```python
from build123d import *

# Parameters (mm, degrees)
SKETCH1_R           = 6.25
BOSS_EXTRUDE1_DEPTH = 8
BOSS_EXTRUDE1_DRAFT = -3
BOSS_EXTRUDE2_DEPTH = 4.5
SKETCH3_R           = 5
BOSS_EXTRUDE3_DEPTH = 2
SKETCH9_R           = 3.5
BOSS_EXTRUDE6_DEPTH = 0.5
FILLET1_R           = 1
SKETCH4_R           = 3
BOSS_EXTRUDE4_DEPTH = 1
SKETCH5_R           = 5
BOSS_EXTRUDE5_DEPTH = 2
SKETCH6_R           = 2
CUT_EXTRUDE1_DEPTH  = 9.5
CUT_EXTRUDE2_DEPTH  = 6.5
SKETCH8_R           = 4.5
CUT_EXTRUDE3_DEPTH  = 2


with BuildPart() as part:
    # Sketch1 → Boss-Extrude1 (with draft: the straight prism first)
    with BuildSketch(Plane.XY):
        Circle(SKETCH1_R)
    extrude(amount=BOSS_EXTRUDE1_DEPTH)
    # Boss-Extrude1: the draft: its side faces are tilted about the plane it starts from
    boss_extrude1_sides = [part.faces().sort_by_distance(p)[0] for p in [
        (-6.25, 0, 4),
    ]]
    draft(boss_extrude1_sides, Plane.XY, BOSS_EXTRUDE1_DRAFT)

    # Sketch2 → Boss-Extrude2 (add)
    with BuildSketch(Plane.XY.offset(8)):
        Polygon((8.082903769, 0), (4.041451884, 7), (-4.041451884, 7), (-8.082903769, 0), (-4.041451884, -7), (4.041451884, -7), align=None)
    extrude(amount=BOSS_EXTRUDE2_DEPTH)

    # Sketch3 → Boss-Extrude3 (add)
    with BuildSketch(Plane.XY.offset(12.5)):
        Circle(SKETCH3_R)
    extrude(amount=BOSS_EXTRUDE3_DEPTH)

    # Sketch9 → Boss-Extrude6 (add)
    with BuildSketch(Plane.XY.offset(14.5)):
        Circle(SKETCH9_R)
    extrude(amount=BOSS_EXTRUDE6_DEPTH)

    # Fillet1
    fillet1_edges = [part.edges().sort_by_distance(p)[0] for p in [
        (-5, 0, 14.5),
    ]]
    fillet(fillet1_edges, radius=FILLET1_R)

    # Sketch4 → Boss-Extrude4 (add)
    with BuildSketch(Plane.XY.offset(15)):
        Circle(SKETCH4_R)
    extrude(amount=BOSS_EXTRUDE4_DEPTH)

    # Sketch5 → Boss-Extrude5 (add)
    with BuildSketch(Plane.XY.offset(16)):
        Circle(SKETCH5_R)
    extrude(amount=BOSS_EXTRUDE5_DEPTH)

    # Sketch6 → Cut-Extrude1 (cut)
    with BuildSketch(Plane.XY.offset(18)):
        Circle(SKETCH6_R)
    extrude(amount=-CUT_EXTRUDE1_DEPTH, mode=Mode.SUBTRACT)

    # Sketch7 → Cut-Extrude2 (cut)
    with BuildSketch(Plane.XY.offset(8.5)):
        Polygon((0, -1.732050808), (1.5, -0.866025404), (1.5, 0.866025404), (0, 1.732050808), (-1.5, 0.866025404), (-1.5, -0.866025404), align=None)
    extrude(amount=-CUT_EXTRUDE2_DEPTH, mode=Mode.SUBTRACT)

    # Sketch8 → Cut-Extrude3 (cut)
    with BuildSketch(Plane(origin=(0, 0, 0), x_dir=(-1, 0, 0), z_dir=(0, 0, -1))):
        Circle(SKETCH8_R)
    extrude(amount=-CUT_EXTRUDE3_DEPTH, mode=Mode.SUBTRACT)


solid = part.part
```
Check sheet for the modelled part. Datum: model origin and axes. Units: mm. A direction names the side the tool comes from. Give positions to 0.01 mm unless a question says otherwise; leave off trailing zeros. Write each loop counter-clockwise with the first axis right and the second up, starting at its lowest first coordinate (ties: lowest second). Pieces come first, ordered by that corner, then holes. Notation, with made-up numbers: (44.25, 15.25) - (99.25, 15.25) arc R15 cw to (99.25, 27.25) - close; hole circle Ø2 at (53, 35.5). An arc over 180 degrees is marked (long way). Answer as a JSON object with one key per item and string values. Group by question number.
1) Access from +Z, -Z, +X, -X, +Y, -Y to the whole of each face (thin tool, end or side, straight path). Record for faces 1 (the face through (6.09, 3.45, 10.22)), 2 (the face through (3, 1, 15)), 3 (the face through (-0.76, -1.293, 5.296)), 4 (the face through (0, -2, 2)), 5 (the face through (0, -2, 13)).
2) Sectioned sample at A-A (z = 10.25). Record the cut outline in (x, y).
3) Thickness scan on probe 1 along Z at (x, y) = (-3, 2); probe 2 along Z at (x, y) = (4.25, 1.75); probe 3 along Y at (x, z) = (0, 11.5). Record the ranges inside material, lowest first. Write a range as from..to.
4) Release check for a two-part mould opening along Z. For faces 6 (the face through (2, 5, 12.5)), 7 (the face through (-3, 0.1, 15.5)), 8 (the face through (0.59, 4.46, 0.99)) record: pulls with the +Z half, pulls with the -Z half, needs draft (parallel to the pull), parting line crosses it, or undercut.
5) Sectioned sample at D-D (z = 1.75). Record the cut outline in (x, y).
6) Sectioned sample at B-B (x = 7). Record the cut outline in (y, z), then the cut area to 3 significant figures.
7) Sectioned sample at C-C (z = 13.75). Record the cut outline in (x, y), then the cut area to 3 significant figures.
8) Depth check by flat-ended pin: P1, Ø3.5, axis at x = -1.5, y = -0.5, coming from the +Z side; P2, Ø1.5, axis at x = -5, y = -5, coming from the +Z side; P3, Ø0.9, axis at y = -0.5, z = 4, coming from the +X side; P4, Ø6.5, axis at x = 0, y = 0, coming from the -Z side. Enter the tip coordinate at first touch or a pass-through.
Geometry results:
{
 "1": {"face 1": "+Z, -Z, +X, +Y", "face 2": "none", "face 3": "+Z, -Z", "face 4": "-Z", "face 5": "+Z"},
 "2": {"outline": "(-8.08, 0) - (-4.04, -7) - (4.04, -7) - (8.08, 0) - (4.04, 7) - (-4.04, 7) - close; hole circle Ø4 at (0, 0)"},
 "3": {"probe 1": "z = 2..14.5, 16..18", "probe 2": "z = 0..14.3, 16..18", "probe 3": "y = -7..-2, 2..7"},
 "4": {"face 6": "pulls with the +Z half", "face 7": "undercut", "face 8": "needs draft"},
 "5": {"outline": "circle Ø12.68 at (0, 0); hole circle Ø9 at (0, 0)"},
 "6": {"outline": "(-1.88, 8) - (1.88, 8) - (1.88, 12.5) - (-1.88, 12.5) - close", "area": "16.9 mm^2"},
 "7": {"outline": "circle Ø9.94 at (0, 0); hole circle Ø4 at (0, 0)", "area": "65.0 mm^2"},
 "8": {"P1": "stops at z = 18", "P2": "stops at z = 12.5", "P3": "stops at x = 6.47", "P4": "stops at z = 2"}
}
